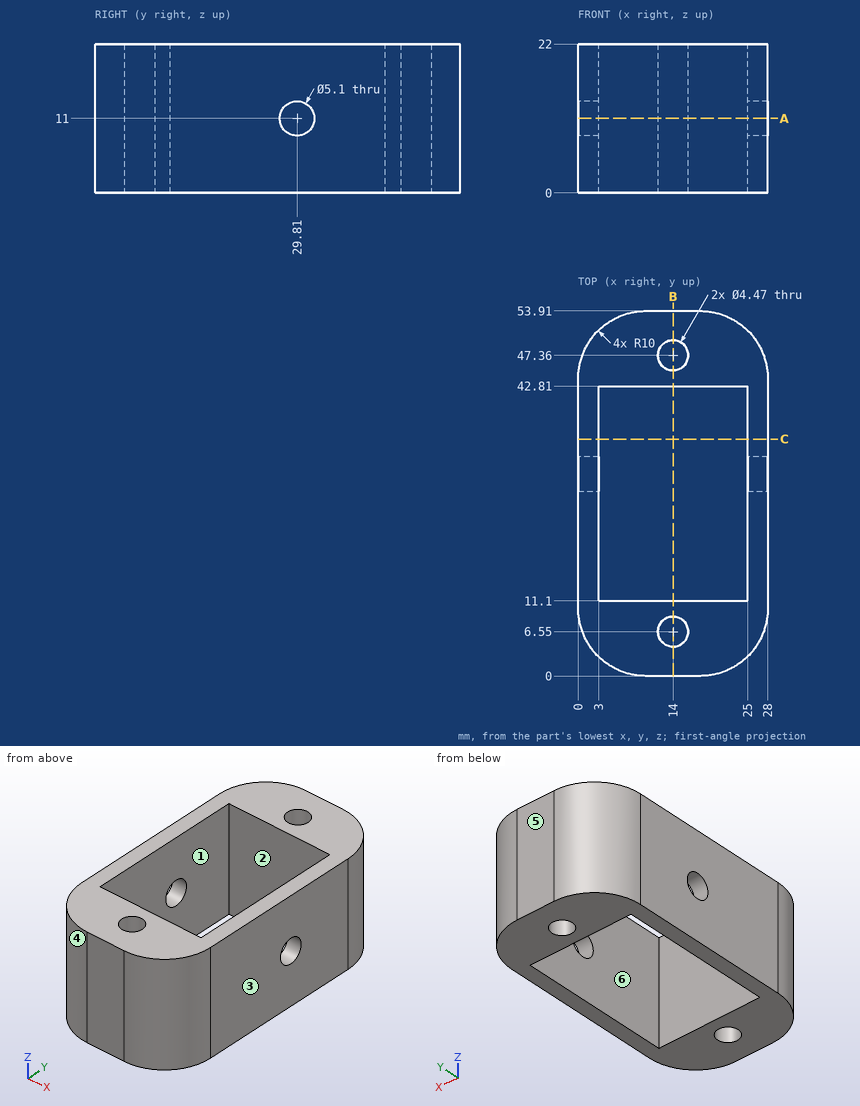
Here's the drawing with two shaded views (mm, measured from the low corner). I have some questions. A direction names the side the tool comes from. Round coordinates to 2 decimals unless told otherwise and drop trailing zeros. Order: outer loops, then holes, each group sorted by start corner. A loop starts at its lowest first (then second) coordinate and runs counter-clockwise, first axis right, second up. Notation, with made-up numbers: M 51,15.5 L 62,15.5 A29 ccw 62,39.5 Z; hole C 71,-33.75 d10. An arc over 180 degrees is marked long. Use CSV: the item, a comma, the result in double quotes.
1) If we mould it in two halves opening along Y, with no side actions, what happens to the marked faces 1, 2, 3 and 4? For each: pulls with the +Y half, pulls with the -Y half, needs draft (parallel to the pull), parting line crosses it, or undercut.
Taken from the geometry:
face 1,"undercut"
face 2,"undercut"
face 3,"needs draft"
face 4,"pulls with the -Y half"
2) I want a section at C-C (y = 35). List the corners of the cut face in (x, z) for me, then the cut area to 3 significant figures.
Taken from the geometry:
outline,"M 0,0 L 3,0 L 3,22 L 0,22 Z; M 25,0 L 28,0 L 28,22 L 25,22 Z"
area,"132 mm^2"
3) I'm going to push a flat-ended pin straight in: P1, Ø4, axis at x = 14, y = 47.36, coming from the -Z side. Where does the tip first touch, or does it pass through?
Taken from the geometry:
P1,"through"
4) I need wall thicknesses on line 1 along Y through (x, z) = (14, 14) (1 decimal); line 2 along Y through (x, z) = (16.5, 12.5); line 3 along Z through (x, y) = (27, 29.81). Which ranges of each line are inside material? Lowest first, please. Write a range as [from, to].
Taken from the geometry:
line 1,"[0, 4.3], [8.8, 11.1], [42.8, 45.1], [49.6, 53.9]"
line 2,"[0, 11.1], [42.81, 53.91]"
line 3,"[0, 8.45], [13.55, 22]"
5) I want a section at B-B (x = 14). List the corners of the cut face in (y, z) for me (1 decimal), then the cut area to 3 significant figures.
Taken from the geometry:
outline,"M 0,0 L 4.3,0 L 4.3,22 L 0,22 Z; M 8.8,0 L 11.1,0 L 11.1,22 L 8.8,22 Z; M 42.8,0 L 45.1,0 L 45.1,22 L 42.8,22 Z; M 49.6,0 L 53.9,0 L 53.9,22 L 49.6,22 Z"
area,"292 mm^2"
6) On a 3-axis mill with a long thin cutter (end or side, diameter ignored), from which of +Z, -Z, +X, -X, +Y, -Y can I reach the whole of each face in a straight line? I mean the marked faces 5 and 6. Say none if no direction works.
Taken from the geometry:
face 5,"+Z, -Z, +X, -X, +Y"
face 6,"+Z, -Z"
7) I want a section at A-A (z = 11). Count the separate pieces of the cut face and the enclosed holes in it, then the cut area to 3 significant figures.
Taken from the geometry:
separate pieces,"2"
enclosed holes,"2"
area,"664 mm^2"
